```python
from build123d import *
from OCP.BRepFilletAPI import BRepFilletAPI_MakeChamfer

# Parameters (mm, degrees)
SKETCH1_W           = 200
SKETCH1_H           = 200
BOSS_EXTRUDE1_DEPTH = 70
FILLET1_R           = 20
FILLET2_R           = 2
SKETCH2_W           = 230.455547831
SKETCH2_H           = 230.807926345
CUT_EXTRUDE1_DEPTH  = 1
SKETCH3_R           = 2.5
CUT_EXTRUDE2_DEPTH  = 5
CHAMFER1_SIZE       = 0.5
CHAMFER1_SIZE2      = 0.288675135
CHAMFER2_SIZE       = 0.5
CHAMFER2_SIZE2      = 0.288675135


with BuildPart() as part:
    # Sketch1 → Boss-Extrude1 (new body)
    with BuildSketch(Plane.XY):
        with Locations((100, 100)):
            Rectangle(SKETCH1_W, SKETCH1_H)
    extrude(amount=BOSS_EXTRUDE1_DEPTH)

    # Fillet1
    fillet1_edges = [part.edges().sort_by_distance(p)[0] for p in [
        (0, 0, 35),
        (200, 0, 35),
        (200, 200, 35),
        (0, 200, 35),
    ]]
    fillet(fillet1_edges, radius=FILLET1_R)

    # Fillet2
    fillet2_edges = [part.edges().sort_by_distance(p)[0] for p in [
        (100, 200, 0),
        (100, 200, 70),
        (0, 100, 0),
        (200, 100, 0),
        (100, 0, 0),
        (5.857864376, 5.857864376, 0),
        (5.857864376, 194.142135624, 0),
        (194.142135624, 5.857864376, 0),
        (194.142135624, 194.142135624, 0),
        (200, 100, 70),
        (0, 100, 70),
        (100, 0, 70),
        (5.857864376, 5.857864376, 70),
        (5.857864376, 194.142135624, 70),
        (194.142135624, 5.857864376, 70),
        (194.142135624, 194.142135624, 70),
    ]]
    fillet(fillet2_edges, radius=FILLET2_R)

    # Sketch2 → Cut-Extrude1 (cut)
    with BuildSketch(Plane(origin=(0, 0, 10), x_dir=(-1, 0, 0), z_dir=(0, 0, -1))):
        with Locations((-100.412379168, 99.554731442)):
            Rectangle(SKETCH2_W, SKETCH2_H)
        with BuildLine():
            Line((-7, 20), (-7, 180))
            ThreePointArc((-7, 180), (-10.807611845, 189.192388155), (-20, 193))
            Line((-20, 193), (-180, 193))
            ThreePointArc((-180, 193), (-189.192388155, 189.192388155), (-193, 180))
            Line((-193, 180), (-193, 20))
            ThreePointArc((-193, 20), (-189.192388155, 10.807611845), (-180, 7))
            Line((-180, 7), (-20, 7))
            ThreePointArc((-20, 7), (-10.807611845, 10.807611845), (-7, 20))
        make_face(mode=Mode.SUBTRACT)
    extrude(amount=-CUT_EXTRUDE1_DEPTH, mode=Mode.SUBTRACT)

    # Sketch3 → Cut-Extrude2 (cut)
    with BuildSketch(Plane.ZY):
        with Locations((6, 125)):
            Circle(SKETCH3_R)
        with Locations((6, 75)):
            Circle(SKETCH3_R)
    cut_extrude2 = extrude(amount=-CUT_EXTRUDE2_DEPTH, mode=Mode.SUBTRACT)

    # Chamfer1
    chamfer1_edges = [part.edges().sort_by_distance(p)[0] for p in [
        (0, 125, 3.5),
        (0, 75, 3.5),
    ]]
    chamfer1_side = [part.faces().sort_by_distance(p)[0] for p in [
        (0, 100, 6),
    ]]
    chamfer(chamfer1_edges, length=CHAMFER1_SIZE, length2=CHAMFER1_SIZE2, reference=chamfer1_side[0])

    # Mirror2: Cut-Extrude2 across plane
    add(cut_extrude2.mirror(Plane.ZY.offset(-100)), mode=Mode.SUBTRACT)

    # Chamfer2: one chamfer whose edges measure the first distance from different faces: ONE call of the kernel's chamfer builder (chamfer() names one face for all edges)
    chamfer2_edges_1 = [part.edges().sort_by_distance(p)[0] for p in [
        (200, 125, 3.5),
    ]]
    chamfer2_side_1 = [part.faces().sort_by_distance(p)[0] for p in [
        (197.5, 125, 3.5),
    ]]
    chamfer2_edges_2 = [part.edges().sort_by_distance(p)[0] for p in [
        (200, 75, 3.5),
    ]]
    chamfer2_side_2 = [part.faces().sort_by_distance(p)[0] for p in [
        (197.5, 75, 3.5),
    ]]
    chamfer2 = BRepFilletAPI_MakeChamfer(part.part.solid().wrapped)
    for e in chamfer2_edges_1:
        chamfer2.Add(CHAMFER2_SIZE, CHAMFER2_SIZE2, e.wrapped, chamfer2_side_1[0].wrapped)  # the first distance lies on this face
    for e in chamfer2_edges_2:
        chamfer2.Add(CHAMFER2_SIZE, CHAMFER2_SIZE2, e.wrapped, chamfer2_side_2[0].wrapped)  # the first distance lies on this face
    add(Compound.cast(chamfer2.Shape()), mode=Mode.REPLACE)


solid = part.part
```
Could you check a few things on this model? Use its own coordinates, in mm. A direction names the side the tool comes from. Give positions to 0.01 mm unless a question says otherwise; leave off trailing zeros.
Q1. If I drill on line 1 along Y through (x, z) = (197.55, 6); line 2 along Y through (x, z) = (196, 6); line 3 along Y through (x, z) = (17, 29), over which ranges is the centre line in solid material (lowest first)?
Q2. I'm going to push flat-ended pins straight in: P1, Ø3, axis at y = 125, z = 6, coming from the +X side; P2, Ø0.5, axis at y = 89, z = 10.5, coming from the +X side; P3, Ø1.5, axis at y = 74, z = 7, coming from the -X side. Where does each tip first touch, or does it pass through?
Q3. We'd pull the mould along Y, two halves only. Please class faces 6 (the flat face through (5, 75, 6)), 7 (the cylindrical face through (194.297, 193.986, 39.899)), 8 (the flat face through (200, 99, 39)): +Y half, -Y half, draft (parallel to the pull), parting line (faces both ways), or undercut.
Q4. For faces 1 (the flat face through (5, 125, 6)), 2 (the cylindrical face through (10.707, 189.091, 10.493)), 3 (the flat face through (197, 100, 10)), 4 (the cylindrical face through (193.986, 5.703, 6.056)), 5 (the flat face through (0, 99, 39)), which set-ups out of +Z, -Z, +X, -X, +Y, -Y let a thin tool reach every point of the face, with its end or its side?
Solution:
1. line 1: y = 10.41 to 72.5, 77.5 to 122.5, 127.5 to 189.59
1. line 2: y = 8 to 72.5, 77.5 to 122.5, 127.5 to 192
1. line 3: y = 0.23 to 199.77
2. P1: stops at x = 195
2. P2: stops at x = 193
2. P3: stops at x = 5
3. face 6: undercut
3. face 7: +Y half
3. face 8: draft
4. face 1: -X
4. face 2: -X, +Y
4. face 3: none
4. face 4: +Z, -Z, +X, -Y
4. face 5: +Z, -Z, -X, +Y, -Y
